Study the drawing (mm; zero at the part's minimum x, y, z) and answer. A direction names the side the tool comes from. Round coordinates to 2 decimals unless told otherwise and drop trailing zeros. Loops run counter-clockwise (first coordinate to the right, second up) from the corner with the lowest first, then second, coordinate; pieces in that order, holes last. Notation, with made-up numbers: (-27.75, 10.25) - (24.25, 10.25) arc R11 cw to (24.25, 20.25) - close; hole circle Ø6 at (85.25, 5). An arc over 180 degrees is marked (long way). One line per item, written item: value.
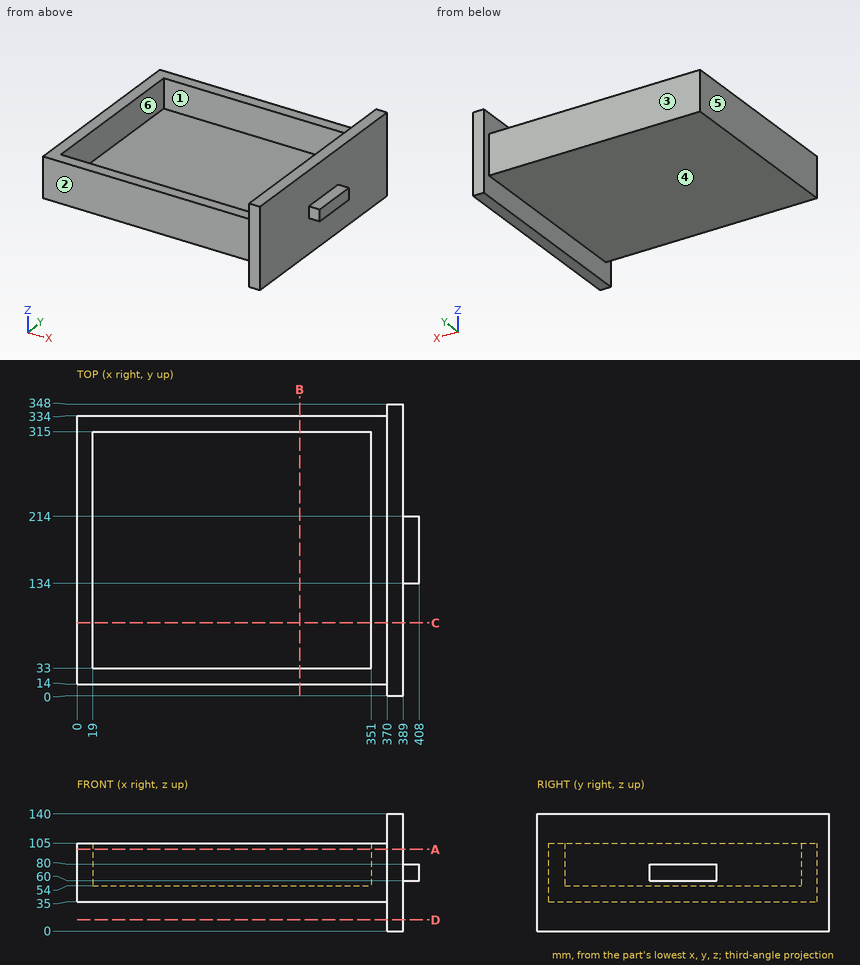
1) A cutting plane is placed at D-D on z = 13.5. Give the vertices of the cut face in (x, y).
Final values:
outline: (370, 0) - (389, 0) - (389, 348) - (370, 348) - close
2) Each of these flat-tipped pins is pushed along its axis until it touches: pin 1 Ø3 at (x, z) = (339.5, 80.5) entering from -Y; pin 2 Ø5.5 at (x, z) = (394.5, 69) entering from +Y; pin 3 Ø21 at (x, z) = (239.5, 85) entering from +Y. Where does it stop, or does it pass through?
Final values:
pin 1: y = 14
pin 2: y = 214
pin 3: y = 334
3) For a pull along X with two mould halves and no side action, classify the marked faces 4, 5 and 6 as released by +X, released by -X, zero draft, split by the parting line, or undercut.
Final values:
face 4: zero draft
face 5: released by -X
face 6: undercut
4) A cutting plane is placed at B-B on x = 265.5. Give the vertices of the cut face in (y, z), and give its area (3 significant figures).
Final values:
outline: (14, 35) - (334, 35) - (334, 105) - (315, 105) - (315, 54) - (33, 54) - (33, 105) - (14, 105) - close
area: 8,020 mm2
5) A cutting plane is placed at C-C on y = 87. Give the vertices of the cut face in (x, z).
Final values:
outline: (0, 35) - (370, 35) - (370, 0) - (389, 0) - (389, 140) - (370, 140) - (370, 105) - (351, 105) - (351, 54) - (19, 54) - (19, 105) - (0, 105) - close
6) Consider L1, parallel to X at y = 200, z = 95.5; L2, parallel to Y at x = 307, z = 98; L3, parallel to X at y = 150, z = 75. Determine where each line is inside the solid, lowest interval first.
Final values:
L1: 0 to 19, 351 to 389
L2: 14 to 33, 315 to 334
L3: 0 to 19, 351 to 408
7) For the marked faces 1, 2 and 3, determine the directions among +Z, -Z, +X, -X, +Y, -Y from which every point of the face is accessible in a straight line to the end or side of a thin tool.
Final values:
face 1: +Z
face 2: +Z, -Z, -X, -Y
face 3: +Z, -Z, -X, +Y
8) A cutting plane is placed at A-A on z = 97.5. Give the vertices of the cut face in (x, y), and give its area (3 significant figures).
Final values:
outline: (0, 14) - (370, 14) - (370, 0) - (389, 0) - (389, 348) - (370, 348) - (370, 334) - (0, 334) - close; hole (19, 33) - (351, 33) - (351, 315) - (19, 315) - close
area: 31,400 mm2
